Answer from the drawing. Dimensions are ordinates in mm from the lowest x, y and z of the part. Give positions to 0.01 mm unless a question says otherwise; leave off trailing zeros. Order: outer loops, then holes, each group sorted by start corner. A loop starts at its lowest first (then second) coordinate and runs counter-clockwise, first axis right, second up.
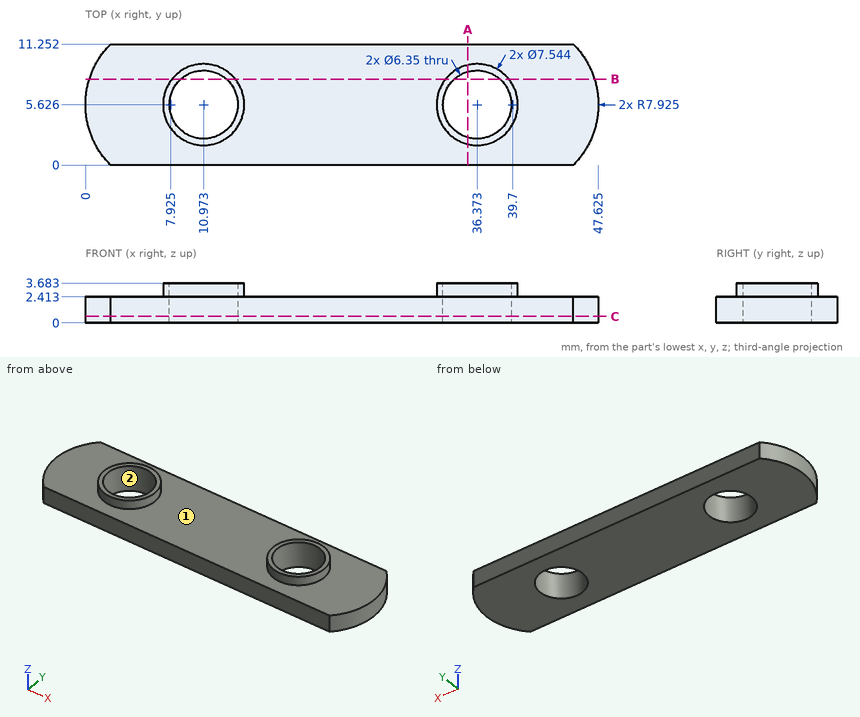
1. The part is cut by section B-B (y = 8). Write down the section's boundary in (x, z), then the cut area to 3 significant figures.
Findings below:
outline: (0.36, 0) - (8.86, 0) - (8.86, 3.68) - (8.04, 3.68) - (8.04, 2.41) - (0.36, 2.41) - close; (13.08, 0) - (34.26, 0) - (34.26, 3.68) - (33.44, 3.68) - (33.44, 2.41) - (13.9, 2.41) - (13.9, 3.68) - (13.08, 3.68) - close; (38.48, 0) - (47.26, 0) - (47.26, 2.41) - (39.3, 2.41) - (39.3, 3.68) - (38.48, 3.68) - close
area: 97.0 mm2
2. Straight lines are drawn through the part: probe 1 along X at (y, z) = (8.5, 1.45) (1 decimal); probe 2 along X at (y, z) = (4, 0.3) (1 decimal); probe 3 along Y at (x, z) = (11, 1.8). For each, find the intervals that lie inside material, in ascending order.
Findings below:
probe 1: x = 0.5 to 9.6, 12.3 to 35, 37.7 to 47.1
probe 2: x = 0.2 to 8.2, 13.7 to 33.6, 39.1 to 47.5
probe 3: y = 0 to 2.45, 8.8 to 11.25
3. Given P1, Ø4, axis at x = 30, y = 2, coming from the +Z side, flat-ended and moving along its own axis, determine where the tip first touches the part or whether it passes through.
Findings below:
P1: stops at z = 2.41
4. The mould has two halves that part along Y. Classify the marked faces 1 and 2: pulls with the +Y half, pulls with the -Y half, needs draft (parallel to the pull), parting line crosses it, or undercut.
Findings below:
face 1: needs draft
face 2: undercut
5. The part is cut by section C-C (z = 0.6). State how many separate pieces and enclosed holes the cut face has, then the cut area to 3 significant figures.
Findings below:
separate pieces: 1
enclosed holes: 2
area: 456 mm2
6. The part is cut by section A-A (x = 35.5). Write down the section's boundary in (y, z).
Findings below:
outline: (0, 0) - (2.57, 0) - (2.57, 3.68) - (1.96, 3.68) - (1.96, 2.41) - (0, 2.41) - close; (8.68, 0) - (11.25, 0) - (11.25, 2.41) - (9.3, 2.41) - (9.3, 3.68) - (8.68, 3.68) - close
